Geometry: final body of the model. Coordinates: model frame, mm. Face numbers are marked on the shaded views. Coordinates: 2 decimals unless noted, no trailing zeros. Loops run counter-clockwise (first coordinate to the right, second up) from the corner with the lowest first, then second, coordinate; pieces in that order, holes last. Notation, with made-up numbers: (3, 75.25) -> (21, 75.25) arc R26 cw to (21, 101.25) -> close; hole circle Ø8 at (41, 89). An arc over 180 degrees is marked (long way). One line per item, written item: value. Start each with the question number.
Item 1: Ray query, probe 1 along X at (y, z) = (7, 0); probe 2 along Z at (x, y) = (0, 6.25); probe 3 along X at (y, z) = (4, 2). Return the intervals inside material, ascending. Write a range as from..to.
Item 2: Section query C-C on z = -1. Return loops of the section in (x, y).
Item 3: Mould query, pull axis X, two halves, no side actions, for the marked faces 1, 2 and 3. Classes: +X half, -X half, draft (parallel to the pull), parting line (faces both ways), or undercut.
Item 4: Section query D-D on y = 7. Return loops of the section in (x, z).
Item 5: Section query B-B on y = 1.5. Return loops of the section in (x, z), then the cut area to 3 significant figures.
Item 6: Section query A-A on x = 15. Return loops of the section in (y, z), then the cut area to 3 significant figures.
Item 7: Contact query for flat-ended pins moving along their axis: pin 1 Ø7 at (x, z) = (0, 0) entering from +Y; pin 2 Ø2 at (x, z) = (0.5, -1.5) entering from -Y; pin 3 Ø4 at (x, z) = (-8, 0) entering from +Y. Output: stop coordinate, or through.
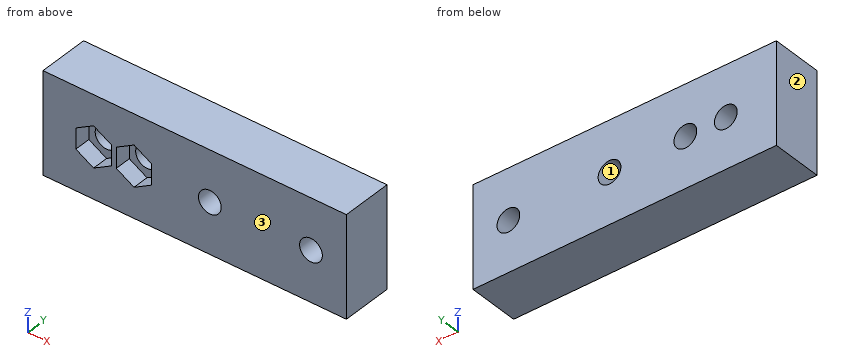
from build123d import *

# Parameters (mm, degrees)
SKETCH1_W           = 60
SKETCH1_H           = 20
SKETCH1_R           = 2.25
BOSS_EXTRUDE1_DEPTH = 10
CUT_EXTRUDE1_DEPTH  = 3.2


with BuildPart() as part:
    # Sketch1 → Boss-Extrude1 (new body)
    with BuildSketch(Plane(origin=(0, 0, 0), x_dir=(1, 0, 0), z_dir=(0, 1, 0))):
        with Locations((12, 0)):
            Rectangle(SKETCH1_W, SKETCH1_H)
        Circle(SKETCH1_R, mode=Mode.SUBTRACT)
        with Locations((-8, 0)):
            Circle(SKETCH1_R, mode=Mode.SUBTRACT)
        with Locations((35, 0)):
            Circle(SKETCH1_R, mode=Mode.SUBTRACT)
        with Locations((15, 0)):
            Circle(SKETCH1_R, mode=Mode.SUBTRACT)
    extrude(amount=BOSS_EXTRUDE1_DEPTH)

    # Sketch2 → Cut-Extrude1 (cut)
    with BuildSketch(Plane.XZ):
        Polygon((-3.5, 2.020725942), (-3.5, -2.020725942), (0, -4.041451884), (3.5, -2.020725942), (3.5, 2.020725942), (0, 4.041451884), align=None)
        Polygon((-4.5, 2.020725942), (-8, 4.041451884), (-11.5, 2.020725942), (-11.5, -2.020725942), (-8, -4.041451884), (-4.5, -2.020725942), align=None)
    extrude(amount=-CUT_EXTRUDE1_DEPTH, mode=Mode.SUBTRACT)


solid = part.part
Reply:
1. probe 1: x = -18..-10.25, -5.75..-2.25, 2.25..12.75, 17.25..32.75, 37.25..42
1. probe 2: z = -10..-2.25, 2.25..10
1. probe 3: x = -18..-9.03, -6.97..-1.03, 1.03..13.97, 16.03..33.97, 36.03..42
2. outline: (-18, 0) -> (-11.5, 0) -> (-11.5, 3.2) -> (-10.02, 3.2) -> (-10.02, 10) -> (-18, 10) -> close; (-5.98, 3.2) -> (-4.5, 3.2) -> (-4.5, 0) -> (-3.5, 0) -> (-3.5, 3.2) -> (-2.02, 3.2) -> (-2.02, 10) -> (-5.98, 10) -> close; (2.02, 3.2) -> (3.5, 3.2) -> (3.5, 0) -> (12.98, 0) -> (12.98, 10) -> (2.02, 10) -> close; (17.02, 0) -> (32.98, 0) -> (32.98, 10) -> (17.02, 10) -> close; (37.02, 0) -> (42, 0) -> (42, 10) -> (37.02, 10) -> close
3. face 1: undercut
3. face 2: -X half
3. face 3: draft
4. outline: (-18, -10) -> (42, -10) -> (42, 10) -> (-18, 10) -> close; hole circle Ø4.5 at (-8, 0); hole circle Ø4.5 at (0, 0); hole circle Ø4.5 at (15, 0); hole circle Ø4.5 at (35, 0)
5. outline: (-18, -10) -> (42, -10) -> (42, 10) -> (-18, 10) -> close; hole (-11.5, -2.02) -> (-8, -4.04) -> (-4.5, -2.02) -> (-4.5, 2.02) -> (-8, 4.04) -> (-11.5, 2.02) -> close; hole (-3.5, -2.02) -> (0, -4.04) -> (3.5, -2.02) -> (3.5, 2.02) -> (0, 4.04) -> (-3.5, 2.02) -> close; hole circle Ø4.5 at (15, 0); hole circle Ø4.5 at (35, 0)
5. area: 1,080 mm²
6. outline: (0, -10) -> (10, -10) -> (10, -2.25) -> (0, -2.25) -> close; (0, 2.25) -> (10, 2.25) -> (10, 10) -> (0, 10) -> close
6. area: 155 mm²
7. pin 1: stops at y = 10
7. pin 2: stops at y = 3.2
7. pin 3: passes through
